from build123d import *

# Parameters (mm, degrees)
F0_R     = 6
F1_DEPTH = 25


with BuildPart() as f1:
    # F0 (on Top) → F1 (new body)
    with BuildSketch(Plane.XY):
        with BuildLine():
            ThreePointArc((-19.032866, -12), (6.245419, -21.615845), (22.5, 0))
            ThreePointArc((22.5, 0), (6.245419, 21.615845), (-19.032866, 12))
            ThreePointArc((-19.032866, 12), (-22.5, 0), (-19.032866, -12))
        make_face()
        with BuildLine():
            ThreePointArc((-19.032866, -12), (-22.5, 0), (-19.032866, 12))
            Line((-19.032866, 12), (-40, 12))
            ThreePointArc((-40, 12), (-52, 0), (-40, -12))
            Line((-40, -12), (-19.032866, -12))
        make_face()
        with Locations((-40, 0)):
            Circle(F0_R, mode=Mode.SUBTRACT)
    extrude(amount=F1_DEPTH)


solid = f1.part
Work out the finished part from the listing and answer in its coordinate system (mm). A direction names the side the tool comes from. Round coordinates to 2 decimals unless told otherwise and drop trailing zeros. Loops run counter-clockwise (first coordinate to the right, second up) from the corner with the lowest first, then second, coordinate; pieces in that order, holes last. Notation, with made-up numbers: (43.5, 33.5) - (67.5, 33.5) arc R12 cw to (67.5, 45.5) - close; hole circle Ø5 at (28, 76.5). An arc over 180 degrees is marked (long way). Use one line per item in the form item = value. Start each with the question number.
(1) Find section B-B on x = -39. Determine the outline of the cut face in (y, z).
(2) Which of the six approach directions +Z, -Z, +X, -X, +Y, -Y give full straight-line access (tool end or side, diameter ignored) to faces 1 (the face through (-52, 0, 12)), 2 (the face through (-30, -12, 12))?
(3) Find section A-A on y = 1. Determine the outline of the cut face in (x, z), and give its area (3 significant figures).
(4) Find section C-C on z = 20.75. Determine the outline of the cut face in (x, y), and give its area (3 significant figures).
(5) Flat-ended cylindrical pins translate along their axes: P1, Ø6.5, axis at x = -25, z = 17.5, coming from the +Y side; P2, Ø1, axis at x = -35, z = 9.5, coming from the -Y side; P3, Ø4, axis at y = -14.5, z = 18.5, coming from the -X side; P4, Ø6, axis at x = -1, y = -9.5, coming from the -Z side. Find the tip coordinate at first contact, or state that the pin passes through.
(6) Determine the mould class of faces 3 (the face through (-29, 12, 12)), 4 (the face through (-7, 0, 0)), 5 (the face through (-46, 0, 12)) for opening direction Y: +Y half, -Y half, draft (parallel to the pull), parting line (faces both ways), or undercut.
(7) Consider line 1 (Y direction, x = -40, z = 10.5); line 2 (Y direction, x = -39, z = 18.75); line 3 (X direction, y = 3, z = 22.5). Determine where each line is inside the solid, lowest interval first.
(8) Find section D-D on x = -21. Determine the outline of the cut face in (y, z).
Answer list:
q1.outline = (-12, 0) - (-5.92, 0) - (-5.92, 25) - (-12, 25) - close; (5.92, 0) - (12, 0) - (12, 25) - (5.92, 25) - close
q2.face_1 = +Z, -Z, -X
q2.face_2 = +Z, -Z, -X, -Y
q3.outline = (-51.96, 0) - (-45.92, 0) - (-45.92, 25) - (-51.96, 25) - close; (-34.08, 0) - (22.48, 0) - (22.48, 25) - (-34.08, 25) - close
q3.area = 1,570 mm^2
q4.outline = (-40, -12) - (-19.03, -12) arc R22.5 ccw to (22.5, 0) arc R22.5 ccw to (-19.03, 12) - (-40, 12) arc R12 ccw to start; hole circle Ø12 at (-40, 0)
q4.area = 2,150 mm^2
q5.P1 = 12
q5.P2 = -12
q5.P3 = -18.71
q5.P4 = 0
q6.face_3 = +Y half
q6.face_4 = draft
q6.face_5 = undercut
q7.line_1 = -12 to -6, 6 to 12
q7.line_2 = -12 to -5.92, 5.92 to 12
q7.line_3 = -51.62 to -45.2, -34.8 to 22.3
q8.outline = (-12, 0) - (12, 0) - (12, 25) - (-12, 25) - close
